Part model, mm, in its own coordinate system. Give positions to 0.01 mm unless a question says otherwise; leave off trailing zeros. Write each loop counter-clockwise with the first axis right and the second up, starting at its lowest first coordinate (ties: lowest second). Pieces come first, ordered by that corner, then holes. Notation, with made-up numbers: (-38, -10) - (-4, -10) arc R8 ccw to (-4, -5) - close; hole circle Ø8 at (45.25, 25). An arc over 180 degrees is marked (long way). Answer as a JSON object with one key per item and string values. Group by question number.
```python
from build123d import *

# Parameters (mm, degrees)
SCHIZZO1_W                   = 450
SCHIZZO1_H                   = 120
ESTRUSIONE_ESTRUSIONE1_DEPTH = 6
TAGLIO_ESTRUSIONE1_DEPTH     = 10
SCHIZZO3_R                   = 2.25
TAGLIO_ESTRUSIONE2_DEPTH     = 10


with BuildPart() as part:
    # Schizzo1 → Estrusione-Estrusione1 (new body)
    with BuildSketch(Plane.XY):
        Rectangle(SCHIZZO1_W, SCHIZZO1_H)
    extrude(amount=ESTRUSIONE_ESTRUSIONE1_DEPTH)

    # Schizzo2 → Taglio-Estrusione1 (cut)
    with BuildSketch(Plane(origin=(0, 0, 0), x_dir=(-1, 0, 0), z_dir=(0, 0, -1))):
        with BuildLine():
            Line((-50, -14), (50, -14))
            ThreePointArc((50, -14), (65, -29), (50, -44))
            Line((50, -44), (-50, -44))
            ThreePointArc((-50, -44), (-65, -29), (-50, -14))
        make_face()
    extrude(amount=-TAGLIO_ESTRUSIONE1_DEPTH, mode=Mode.SUBTRACT)

    # Schizzo3 → Taglio-Estrusione2 (cut)
    with BuildSketch(Plane.XY.offset(6)):
        with Locations((-171, -12)):
            Circle(SCHIZZO3_R)
        with Locations((-171, -30.5)):
            Circle(SCHIZZO3_R)
        with Locations((171, -12)):
            Circle(SCHIZZO3_R)
        with Locations((171, -30.5)):
            Circle(SCHIZZO3_R)
        with Locations((201, 40)):
            Circle(SCHIZZO3_R)
        with Locations((-201, 40)):
            Circle(SCHIZZO3_R)
        with Locations((127, -2)):
            Circle(SCHIZZO3_R)
        with Locations((127, -25)):
            Circle(SCHIZZO3_R)
        with Locations((-127, -2)):
            Circle(SCHIZZO3_R)
        with Locations((-127, -25)):
            Circle(SCHIZZO3_R)
    extrude(amount=-TAGLIO_ESTRUSIONE2_DEPTH, mode=Mode.SUBTRACT)


solid = part.part
```
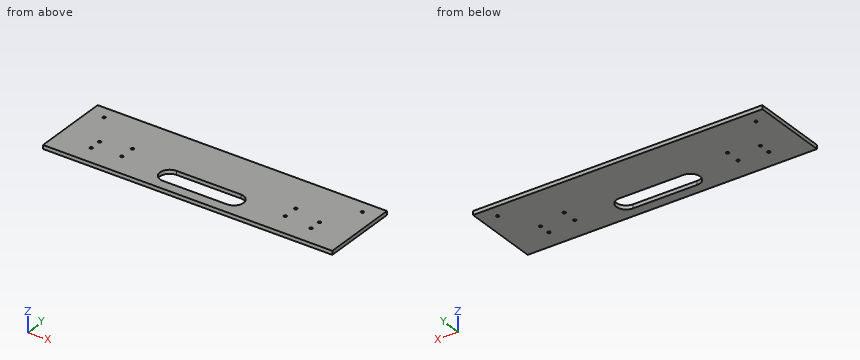
1) Drop a flat-ended pin along its axis: P1, Ø6, axis at x = 171, y = -30.5, coming from the +Z side. Give the stop position or say it passes through.
2) Probe line 1 (Y direction, x = -127, z = 4.05); line 2 (Y direction, x = 171, z = 2); line 3 (X direction, y = -26.5, z = 1.8). List the from-to ranges inside material, lowest first.
3) Band-saw the part on A-A (x = 10). List the corners of the cut face in (y, z).
4) Band-saw the part on B-B (z = 4.9). State how many separate pieces and enclosed holes the cut face has, plus the area to 3 significant figures.
Verdict:
{
 "1": {"P1": "z = 6"},
 "2": {"line 1": "-60 to -27.25, -22.75 to -4.25, 0.25 to 60", "line 2": "-60 to -32.75, -28.25 to -14.25, -9.75 to 60", "line 3": "-225 to -128.68, -125.32 to -64.79, 64.79 to 125.32, 128.68 to 225"},
 "3": {"outline": "(-60, 0) - (-44, 0) - (-44, 6) - (-60, 6) - close; (-14, 0) - (60, 0) - (60, 6) - (-14, 6) - close"},
 "4": {"separate pieces": "1", "enclosed holes": "11", "area": "50,100 mm2"}
}
